```python
from build123d import *

# Parameters (mm, degrees)
F0_W           = 74.5297018439
F0_H           = 75.2062629908
F1_DEPTH       = 25
F6_D           = 13
F6_DEPTH       = 50
F6_CBORE_D     = 22
F6_CBORE_DEPTH = 7.3
F6_TIP         = 3.9055940237


# Not quite as in the source:
# - the program builds the solid bodies; features that only make, move or delete a surface that nothing else refers to are left out


with BuildPart() as f1:
    # F0 (on Front) → F1 (new body)
    with BuildSketch(Plane.XZ):
        with Locations((-55.4675785825, 15.8807532862)):
            Rectangle(F0_W, F0_H)
    extrude(amount=F1_DEPTH)

    # F6
    with Locations(Plane.XZ.offset(25)):
        with Locations((-53.1250275671, 21.3232878596)):
            CounterBoreHole(F6_D / 2, F6_CBORE_D / 2, F6_CBORE_DEPTH, depth=F6_DEPTH)
            with Locations((0, 0, -(F6_DEPTH + F6_TIP / 2))):  # 118° drill point
                Cone(0, F6_D / 2, F6_TIP, mode=Mode.SUBTRACT)


solid = f1.part
```
The model under review builds one solid part; all positions refer to its coordinate system, in mm. A direction names the side the tool comes from. Round coordinates to 2 decimals unless told otherwise and drop trailing zeros. Loops run counter-clockwise (first coordinate to the right, second up) from the corner with the lowest first, then second, coordinate; pieces in that order, holes last.
1) Tool access review of faces 1 (the face through (-56, -12, 53.484)), 2 (the face through (-61.854, -21.401, 14.63)): name each direction out of +Z, -Z, +X, -X, +Y, -Y from which nothing blocks a thin tool from reaching the whole face with its end or side.
Values follow:
face 1: +Z, +X, -X, +Y, -Y
face 2: -Y
2) Clearance check with a flat-ended pin moving along its axis: P1, Ø17.5, axis at x = -53.13, z = 21.32, coming from the -Y side. State where the tip first meets the part, or that it passes through.
Values follow:
P1: stops at y = -17.7
3) Consider section A-A on z = 18. State the section outline as (x, y) points, then the cut area to 3 significant figures.
Values follow:
outline: (-92.73, -25) - (-63.61, -25) - (-63.61, -17.7) - (-58.71, -17.7) - (-58.71, 0) - (-92.73, 0) - close; (-47.54, -17.7) - (-42.64, -17.7) - (-42.64, -25) - (-18.2, -25) - (-18.2, 0) - (-47.54, 0) - close
area: 1,510 mm2
4) Wall thickness on line 1 along Z through (x, y) = (-53, -13.75); line 2 along X through (y, z) = (-6.25, 26); line 3 along X through (y, z) = (-3.5, 27): over which ranges is each line inside the solid? List them lowest first.
Values follow:
line 1: z = -21.72 to 14.82, 27.82 to 53.48
line 2: x = -92.73 to -57.64, -48.61 to -18.2
line 3: x = -92.73 to -56.29, -49.96 to -18.2
5) Consider section B-B on y = -8.25. State the section outline as (x, z) points.
Values follow:
outline: (-92.73, -21.72) - (-18.2, -21.72) - (-18.2, 53.48) - (-92.73, 53.48) - close; hole circle Ø13 at (-53.13, 21.32)
6) The part is to be moulded in two halves that separate along X. For faces 3 (the face through (-46.63, -8.73, 21.61)), 4 (the face through (-48, -17.7, 17)), 5 (the face through (-56, 0, 8)), 6 (the face through (-92.732, -12, 15)), say which applies: pulls with the +X half, pulls with the -X half, needs draft (parallel to the pull), parting line crosses it, or undercut.
Values follow:
face 3: undercut
face 4: undercut
face 5: needs draft
face 6: pulls with the -X half
7) Consider section C-C on z = 26. State the section outline as (x, y) points, then the cut area to 3 significant figures.
Values follow:
outline: (-92.73, -25) - (-63.08, -25) - (-63.08, -17.7) - (-57.64, -17.7) - (-57.64, 0) - (-92.73, 0) - close; (-48.61, -17.7) - (-43.17, -17.7) - (-43.17, -25) - (-18.2, -25) - (-18.2, 0) - (-48.61, 0) - close
area: 1,560 mm2
